```python
from build123d import *

# Parameters (mm, degrees)
F1_DEPTH    = 5
F2_W        = 9
F2_H        = 2.5
F3_DEPTH    = 2.001
F4_T1_DEPTH = 2
F6_DEPTH    = 5.001


# Not quite as in the source:
# - a fillet or chamfer that OpenCascade refuses, or shapes differently, is made with other operations: its cross-section is extruded or revolved along the edge and cut away or added


with BuildPart() as f1:
    # F0 (on Top) → F1 (new body)
    with BuildSketch(Plane.XY):
        with BuildLine():
            Line((5, 1), (-5, 1))
            ThreePointArc((-5, 1), (-5.6464466094, 0.6464466094), (-6, 0))
            ThreePointArc((-6, 0), (-5.6464466094, -0.6464466094), (-5, -1))
            Line((-5, -1), (5, -1))
            ThreePointArc((5, -1), (5.6464466094, -0.6464466094), (6, 0))
            ThreePointArc((6, 0), (5.6464466094, 0.6464466094), (5, 1))
        make_face()
    extrude(amount=F1_DEPTH)

    # F2 (on face) → F3 (cut, through all)
    with BuildSketch(Plane.XZ.offset(1)):
        with Locations((0, 3)):
            Rectangle(F2_W, F2_H)
    extrude(amount=-F3_DEPTH, mode=Mode.SUBTRACT)

    # F4: fillet of radius 1.3 on 4 edges, made by hand

    # F4_s2 → F4_t1 (join)
    with BuildSketch(Plane.XZ.offset(-1)):
        with BuildLine():
            ThreePointArc((-4.5, 3.05), (-4.1192388155, 2.1307611845), (-3.2, 1.75))
            Line((-3.2, 1.75), (-4.5, 1.75))
            Line((-4.5, 1.75), (-4.5, 3.05))
        make_face()
        with BuildLine():
            ThreePointArc((-3.2, 4.25), (-4.1192388155, 3.8692388155), (-4.5, 2.95))
            Line((-4.5, 2.95), (-4.5, 4.25))
            Line((-4.5, 4.25), (-3.2, 4.25))
        make_face()
        with BuildLine():
            ThreePointArc((3.2, 4.25), (4.1192388155, 3.8692388155), (4.5, 2.95))
            Line((4.5, 2.95), (4.5, 4.25))
            Line((4.5, 4.25), (3.2, 4.25))
        make_face()
        with BuildLine():
            ThreePointArc((3.2, 1.75), (4.1192388155, 2.1307611845), (4.5, 3.05))
            Line((4.5, 3.05), (4.5, 1.75))
            Line((4.5, 1.75), (3.2, 1.75))
        make_face()
    extrude(amount=F4_T1_DEPTH)

    # F5 (on face) → F6 (cut, through all)
    with BuildSketch(Plane.XY.offset(5)):
        with BuildLine():
            Line((-4.8, -1), (-4.8, 1))
            Line((-4.8, 1), (-5, 1))
            ThreePointArc((-5, 1), (-5.6464466094, 0.6464466094), (-6, 0))
            ThreePointArc((-6, 0), (-5.6464466094, -0.6464466094), (-5, -1))
            Line((-5, -1), (-4.8, -1))
        make_face()
    extrude(amount=-F6_DEPTH, mode=Mode.SUBTRACT)


solid = f1.part
```
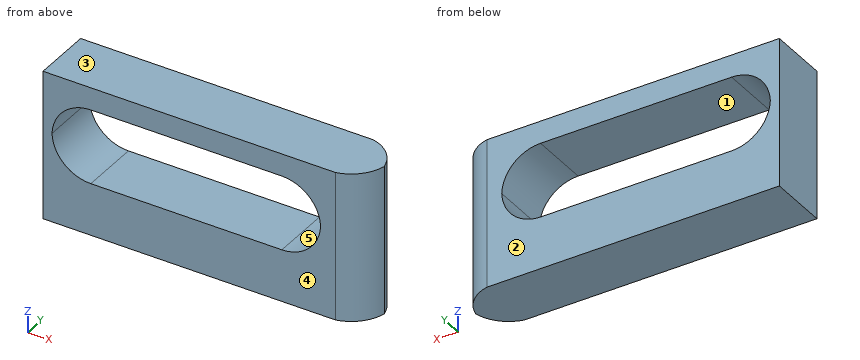
Design review of the part built by this model. Coordinates are the model's own, in mm. Face numbers are marked on the shaded views. A direction names the side the tool comes from. Coordinates: 2 decimals unless noted, no trailing zeros. Order: outer loops, then holes, each group sorted by start corner. A loop starts at its lowest first (then second) coordinate and runs counter-clockwise, first axis right, second up. Notation, with made-up numbers: (14.25, 64.25) -> (27.25, 64.25) arc R33 ccw to (27.25, 101.25) -> close; hole circle Ø9 at (14, 74). An arc over 180 degrees is marked (long way). One line per item, written item: value. Start each with the question number.
Q1. Take a section at C-C, the plane y = -0.2. State the section outline as (x, z) points.
Q2. Mouldability with a two-part tool opening along Z and no side actions: class the marked faces 3, 4 and 5 as pulls with the +Z half, pulls with the -Z half, needs draft (parallel to the pull), parting line crosses it, or undercut.
Q3. For probe 1 along Z at (x, y) = (0.75, 0); probe 2 along X at (y, z) = (0.9, 3.25); probe 3 along X at (y, z) = (-0.6, 3.7), list the stretches that pass through material, from the lowest coordinate up.
Q4. Take a section at A-A, the plane x = 3. State the section outline as (y, z) points.
Q5. Take a section at B-B, the plane z = 2.35. State the section outline as (x, y) points, then the cut area to 3 significant figures.
Q6. Tool access review of the marked faces 1 and 2: name each direction out of +Z, -Z, +X, -X, +Y, -Y from which nothing blocks a thin tool from reaching the whole face with its end or side.
Q7. Take a section at D-D, the plane z = 1.2. State the section outline as (x, y) points, then the cut area to 3 significant figures.
Values follow:
1. outline: (-4.8, 0) -> (5.94, 0) -> (5.94, 5) -> (-4.8, 5) -> close; hole (-4.5, 3) arc R1.3 ccw to (-3.2, 1.75) -> (3.2, 1.75) arc R1.3 ccw to (4.5, 3) arc R1.3 ccw to (3.2, 4.25) -> (-3.2, 4.25) arc R1.3 ccw to start
2. face 3: pulls with the +Z half
2. face 4: needs draft
2. face 5: undercut
3. probe 1: z = 0 to 1.75, 4.25 to 5
3. probe 2: x = -4.8 to -4.46, 4.46 to 5.29
3. probe 3: x = -4.8 to -4.26, 4.26 to 5.69
4. outline: (-1, 0) -> (1, 0) -> (1, 1.75) -> (-1, 1.75) -> close; (-1, 4.25) -> (1, 4.25) -> (1, 5) -> (-1, 5) -> close
5. outline: (-4.8, -1) -> (-4.3, -1) -> (-4.3, 1) -> (-4.8, 1) -> close; (4.3, -1) -> (5, -1) arc R1.31 ccw to (6, 0) arc R1.31 ccw to (5, 1) -> (4.3, 1) -> close
5. area: 3.82 mm2
6. face 1: +Y, -Y
6. face 2: +Z, -Z, +X, -X, +Y
7. outline: (-4.8, -1) -> (5, -1) arc R1.31 ccw to (6, 0) arc R1.31 ccw to (5, 1) -> (-4.8, 1) -> close
7. area: 21.0 mm2
